```python
from build123d import *

# Parameters (mm, degrees)
BOSS_EXTRUDE1_DEPTH = 6.35
BOSS_EXTRUDE2_DEPTH = 6.35
CUT_EXTRUDE2_REACH  = 173.121
SKETCH3_R           = 25.4
SKETCH3_R_2         = 14.2875


with BuildPart() as part:
    # Sketch1 → Boss-Extrude1 (new body)
    with BuildSketch(Plane(origin=(0, 0, 0), x_dir=(1, 0, 0), z_dir=(0, 1, 0))):
        with BuildLine():
            Line((-82.55, -44.45), (-10.295626201, -144.494517568))
            ThreePointArc((-10.295626201, -144.494517568), (0, -149.758787534), (10.295626201, -144.494517568))
            Line((10.295626201, -144.494517568), (82.55, -44.45))
            Line((82.55, -44.45), (82.55, 44.45))
            Line((82.55, 44.45), (-82.55, 44.45))
            Line((-82.55, 44.45), (-82.55, -44.45))
        make_face()
    extrude(amount=BOSS_EXTRUDE1_DEPTH)

    # Sketch4 → Boss-Extrude2 (add)
    with BuildSketch(Plane(origin=(0, 6.35, 0), x_dir=(1, 0, 0), z_dir=(0, 1, 0))):
        Polygon((-63.5, -70.826923077), (-63.5, -96.226923077), (-57.15, -96.226923077), (-57.15, -79.619230769), align=None)
        Polygon((57.15, -96.226923077), (63.5, -96.226923077), (63.5, -70.826923077), (57.15, -79.619230769), align=None)
    extrude(amount=-BOSS_EXTRUDE2_DEPTH)

    # Sketch3 → Cut-Extrude2 (cut, up to next)
    with BuildSketch(Plane(origin=(0, 6.35, 0), x_dir=(1, 0, 0), z_dir=(0, 1, 0)), mode=Mode.PRIVATE) as cut_extrude2_sk1:
        with Locations(Location((0, -50.8, 0), (0, 0, 270))):
            Circle(SKETCH3_R)
    cut_extrude2_tool1 = extrude(cut_extrude2_sk1.sketch, amount=-CUT_EXTRUDE2_REACH, mode=Mode.PRIVATE) & part.part
    # Sketch3 → Cut-Extrude2 (cut, up to next)
    with BuildSketch(Plane(origin=(0, 6.35, 0), x_dir=(1, 0, 0), z_dir=(0, 1, 0)), mode=Mode.PRIVATE) as cut_extrude2_sk2:
        with Locations(Location((0, -120.65, 0), (0, 0, 270))):
            Circle(SKETCH3_R_2)
    cut_extrude2_tool2 = extrude(cut_extrude2_sk2.sketch, amount=-CUT_EXTRUDE2_REACH, mode=Mode.PRIVATE) & part.part
    # Sketch3 → Cut-Extrude2 (cut, up to next)
    with BuildSketch(Plane(origin=(0, 6.35, 0), x_dir=(1, 0, 0), z_dir=(0, 1, 0)), mode=Mode.PRIVATE) as cut_extrude2_sk3:
        with BuildLine():
            Line((-40.026450178, 28.764752129), (-8.690133469, 11.891350824))
            ThreePointArc((-8.690133469, 11.891350824), (-7.123451286, 11.92620437), (-6.35, 13.289098695))
            Line((-6.35, 13.289098695), (-6.35, 30.1625))
            ThreePointArc((-6.35, 30.1625), (-6.814967985, 31.285032015), (-7.9375, 31.75))
            Line((-7.9375, 31.75), (-39.273816708, 31.75))
            ThreePointArc((-39.273816708, 31.75), (-40.813147894, 30.550592453), (-40.026450178, 28.764752129))
        make_face()
    cut_extrude2_tool3 = extrude(cut_extrude2_sk3.sketch, amount=-CUT_EXTRUDE2_REACH, mode=Mode.PRIVATE) & part.part
    # Sketch3 → Cut-Extrude2 (cut, up to next)
    with BuildSketch(Plane(origin=(0, 6.35, 0), x_dir=(1, 0, 0), z_dir=(0, 1, 0)), mode=Mode.PRIVATE) as cut_extrude2_sk4:
        with BuildLine():
            Line((-69.85, 27.741670535), (-69.85, 7.9375))
            ThreePointArc((-69.85, 7.9375), (-69.385032015, 6.814967985), (-68.2625, 6.35))
            Line((-68.2625, 6.35), (-31.483326149, 6.35))
            ThreePointArc((-31.483326149, 6.35), (-29.943994963, 7.549407547), (-30.73069268, 9.335247871))
            Line((-30.73069268, 9.335247871), (-67.509866531, 29.139418406))
            ThreePointArc((-67.509866531, 29.139418406), (-69.076548714, 29.10456486), (-69.85, 27.741670535))
        make_face()
    cut_extrude2_tool4 = extrude(cut_extrude2_sk4.sketch, amount=-CUT_EXTRUDE2_REACH, mode=Mode.PRIVATE) & part.part
    # Sketch3 → Cut-Extrude2 (cut, up to next)
    with BuildSketch(Plane(origin=(0, 6.35, 0), x_dir=(1, 0, 0), z_dir=(0, 1, 0)), mode=Mode.PRIVATE) as cut_extrude2_sk5:
        with BuildLine():
            Line((7.9375, 31.75), (39.273816708, 31.75))
            ThreePointArc((39.273816708, 31.75), (40.813147894, 30.550592453), (40.026450178, 28.764752129))
            Line((40.026450178, 28.764752129), (8.690133469, 11.891350824))
            ThreePointArc((8.690133469, 11.891350824), (7.123451286, 11.92620437), (6.35, 13.289098695))
            Line((6.35, 13.289098695), (6.35, 30.1625))
            ThreePointArc((6.35, 30.1625), (6.814967985, 31.285032015), (7.9375, 31.75))
        make_face()
    cut_extrude2_tool5 = extrude(cut_extrude2_sk5.sketch, amount=-CUT_EXTRUDE2_REACH, mode=Mode.PRIVATE) & part.part
    # Sketch3 → Cut-Extrude2 (cut, up to next)
    with BuildSketch(Plane(origin=(0, 6.35, 0), x_dir=(1, 0, 0), z_dir=(0, 1, 0)), mode=Mode.PRIVATE) as cut_extrude2_sk6:
        with BuildLine():
            Line((30.73069268, 9.335247871), (67.509866531, 29.139418406))
            ThreePointArc((67.509866531, 29.139418406), (69.076548714, 29.10456486), (69.85, 27.741670535))
            Line((69.85, 27.741670535), (69.85, 7.9375))
            ThreePointArc((69.85, 7.9375), (69.385032015, 6.814967985), (68.2625, 6.35))
            Line((68.2625, 6.35), (31.483326149, 6.35))
            ThreePointArc((31.483326149, 6.35), (29.943994963, 7.549407547), (30.73069268, 9.335247871))
        make_face()
    cut_extrude2_tool6 = extrude(cut_extrude2_sk6.sketch, amount=-CUT_EXTRUDE2_REACH, mode=Mode.PRIVATE) & part.part
    # Sketch3 → Cut-Extrude2 (cut, up to next)
    with BuildSketch(Plane(origin=(0, 6.35, 0), x_dir=(1, 0, 0), z_dir=(0, 1, 0)), mode=Mode.PRIVATE) as cut_extrude2_sk7:
        with BuildLine():
            Line((69.85, -27.741670535), (69.85, -7.9375))
            ThreePointArc((69.85, -7.9375), (69.385032015, -6.814967985), (68.2625, -6.35))
            Line((68.2625, -6.35), (31.483326149, -6.35))
            ThreePointArc((31.483326149, -6.35), (29.943994963, -7.549407547), (30.73069268, -9.335247871))
            Line((30.73069268, -9.335247871), (67.509866531, -29.139418406))
            ThreePointArc((67.509866531, -29.139418406), (69.076548714, -29.10456486), (69.85, -27.741670535))
        make_face()
    cut_extrude2_tool7 = extrude(cut_extrude2_sk7.sketch, amount=-CUT_EXTRUDE2_REACH, mode=Mode.PRIVATE) & part.part
    # Sketch3 → Cut-Extrude2 (cut, up to next)
    with BuildSketch(Plane(origin=(0, 6.35, 0), x_dir=(1, 0, 0), z_dir=(0, 1, 0)), mode=Mode.PRIVATE) as cut_extrude2_sk8:
        with BuildLine():
            Line((-30.73069268, -9.335247871), (-67.509866531, -29.139418406))
            ThreePointArc((-67.509866531, -29.139418406), (-69.076548714, -29.10456486), (-69.85, -27.741670535))
            Line((-69.85, -27.741670535), (-69.85, -7.9375))
            ThreePointArc((-69.85, -7.9375), (-69.385032015, -6.814967985), (-68.2625, -6.35))
            Line((-68.2625, -6.35), (-31.483326149, -6.35))
            ThreePointArc((-31.483326149, -6.35), (-29.943994963, -7.549407547), (-30.73069268, -9.335247871))
        make_face()
    cut_extrude2_tool8 = extrude(cut_extrude2_sk8.sketch, amount=-CUT_EXTRUDE2_REACH, mode=Mode.PRIVATE) & part.part
    # Sketch3 → Cut-Extrude2 (cut, up to next)
    with BuildSketch(Plane(origin=(0, 6.35, 0), x_dir=(1, 0, 0), z_dir=(0, 1, 0)), mode=Mode.PRIVATE) as cut_extrude2_sk9:
        with BuildLine():
            Line((-6.35, -85.142875899), (-6.35, -99.265701316))
            ThreePointArc((-6.35, -99.265701316), (-15.402705776, -104.514096399), (-21.066111407, -113.313128703))
            Line((-21.066111407, -113.313128703), (-61.628371026, -57.15))
            Line((-61.628371026, -57.15), (-34.342875899, -57.15))
            ThreePointArc((-34.342875899, -57.15), (-24.695704333, -75.495704333), (-6.35, -85.142875899))
        make_face()
    cut_extrude2_tool9 = extrude(cut_extrude2_sk9.sketch, amount=-CUT_EXTRUDE2_REACH, mode=Mode.PRIVATE) & part.part
    # Sketch3 → Cut-Extrude2 (cut, up to next)
    with BuildSketch(Plane(origin=(0, 6.35, 0), x_dir=(1, 0, 0), z_dir=(0, 1, 0)), mode=Mode.PRIVATE) as cut_extrude2_sk10:
        with BuildLine():
            Line((6.35, -85.142875899), (6.35, -99.265701316))
            ThreePointArc((6.35, -99.265701316), (15.402705776, -104.514096399), (21.066111407, -113.313128703))
            Line((21.066111407, -113.313128703), (61.628371026, -57.15))
            Line((61.628371026, -57.15), (34.342875899, -57.15))
            ThreePointArc((34.342875899, -57.15), (24.695704333, -75.495704333), (6.35, -85.142875899))
        make_face()
    cut_extrude2_tool10 = extrude(cut_extrude2_sk10.sketch, amount=-CUT_EXTRUDE2_REACH, mode=Mode.PRIVATE) & part.part
    # Sketch3 → Cut-Extrude2 (cut, up to next)
    with BuildSketch(Plane(origin=(0, 6.35, 0), x_dir=(1, 0, 0), z_dir=(0, 1, 0)), mode=Mode.PRIVATE) as cut_extrude2_sk11:
        with BuildLine():
            Line((-19.05, -21.527946348), (-19.05, 0))
            ThreePointArc((-19.05, 0), (0, 5.652946348), (19.05, 0))
            Line((19.05, 0), (19.05, -21.527946348))
            ThreePointArc((19.05, -21.527946348), (0, -15.875), (-19.05, -21.527946348))
        make_face()
    cut_extrude2_tool11 = extrude(cut_extrude2_sk11.sketch, amount=-CUT_EXTRUDE2_REACH, mode=Mode.PRIVATE) & part.part
    # Sketch3 → Cut-Extrude2 (cut, up to next)
    with BuildSketch(Plane(origin=(0, 6.35, 0), x_dir=(1, 0, 0), z_dir=(0, 1, 0)), mode=Mode.PRIVATE) as cut_extrude2_sk12:
        with BuildLine():
            Line((-62.859530994, -44.45), (-35.639286609, -44.45))
            ThreePointArc((-35.639286609, -44.45), (-34.646236712, -44.101050827), (-34.089752409, -43.207608696))
            ThreePointArc((-34.089752409, -43.207608696), (-32.045675665, -36.913665127), (-28.851086957, -31.11827227))
            ThreePointArc((-28.851086957, -31.11827227), (-28.645591226, -30.691776493), (-28.575, -30.223648283))
            Line((-28.575, -30.223648283), (-28.575, -25.256406388))
            ThreePointArc((-28.575, -25.256406388), (-29.348451286, -23.893512063), (-30.915133469, -23.858658517))
            Line((-30.915133469, -23.858658517), (-63.612164463, -41.464752129))
            ThreePointArc((-63.612164463, -41.464752129), (-64.398862179, -43.250592453), (-62.859530994, -44.45))
        make_face()
    cut_extrude2_tool12 = extrude(cut_extrude2_sk12.sketch, amount=-CUT_EXTRUDE2_REACH, mode=Mode.PRIVATE) & part.part
    # Sketch3 → Cut-Extrude2 (cut, up to next)
    with BuildSketch(Plane(origin=(0, 6.35, 0), x_dir=(1, 0, 0), z_dir=(0, 1, 0)), mode=Mode.PRIVATE) as cut_extrude2_sk13:
        with BuildLine():
            Line((28.575, -25.256406388), (28.575, -30.223648283))
            ThreePointArc((28.575, -30.223648283), (28.645591226, -30.691776493), (28.851086957, -31.11827227))
            ThreePointArc((28.851086957, -31.11827227), (32.045675665, -36.913665127), (34.089752409, -43.207608696))
            ThreePointArc((34.089752409, -43.207608696), (34.646236712, -44.101050827), (35.639286609, -44.45))
            Line((35.639286609, -44.45), (62.859530994, -44.45))
            ThreePointArc((62.859530994, -44.45), (64.398862179, -43.250592453), (63.612164463, -41.464752129))
            Line((63.612164463, -41.464752129), (30.915133469, -23.858658517))
            ThreePointArc((30.915133469, -23.858658517), (29.348451286, -23.893512063), (28.575, -25.256406388))
        make_face()
    cut_extrude2_tool13 = extrude(cut_extrude2_sk13.sketch, amount=-CUT_EXTRUDE2_REACH, mode=Mode.PRIVATE) & part.part
    add(cut_extrude2_tool1.solids().sort_by_distance((0, 6.35, 50.8))[0], mode=Mode.SUBTRACT)
    add(cut_extrude2_tool2.solids().sort_by_distance((0, 6.35, 120.65))[0], mode=Mode.SUBTRACT)
    add(cut_extrude2_tool3.solids().sort_by_distance((-19.115543, 6.35, -24.652033))[0], mode=Mode.SUBTRACT)
    add(cut_extrude2_tool4.solids().sort_by_distance((-55.236845, 6.35, -14.418636))[0], mode=Mode.SUBTRACT)
    add(cut_extrude2_tool5.solids().sort_by_distance((19.115543, 6.35, -24.652033))[0], mode=Mode.SUBTRACT)
    add(cut_extrude2_tool6.solids().sort_by_distance((55.236845, 6.35, -14.418636))[0], mode=Mode.SUBTRACT)
    add(cut_extrude2_tool7.solids().sort_by_distance((55.236845, 6.35, 14.418636))[0], mode=Mode.SUBTRACT)
    add(cut_extrude2_tool8.solids().sort_by_distance((-55.236845, 6.35, 14.418636))[0], mode=Mode.SUBTRACT)
    add(cut_extrude2_tool9.solids().sort_by_distance((-30.896348, 6.35, 81.78683))[0], mode=Mode.SUBTRACT)
    add(cut_extrude2_tool10.solids().sort_by_distance((30.896348, 6.35, 81.78683))[0], mode=Mode.SUBTRACT)
    add(cut_extrude2_tool11.solids().sort_by_distance((0, 6.35, 6.929783))[0], mode=Mode.SUBTRACT)
    add(cut_extrude2_tool12.solids().sort_by_distance((-43.155831, 6.35, 36.82378))[0], mode=Mode.SUBTRACT)
    add(cut_extrude2_tool13.solids().sort_by_distance((43.155831, 6.35, 36.82378))[0], mode=Mode.SUBTRACT)


solid = part.part
```
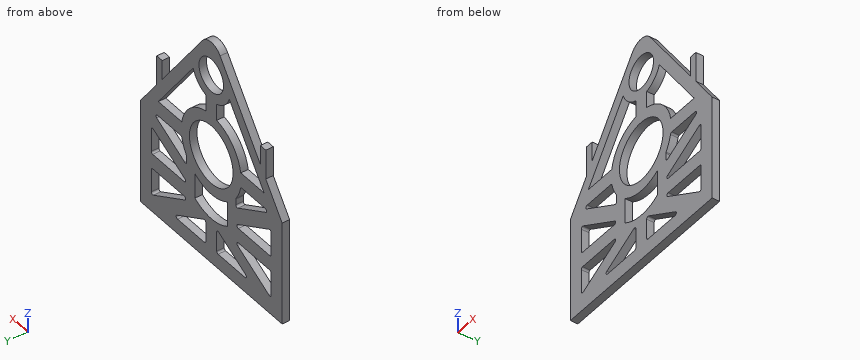
Input: part model. Units: mm. Frame: model coordinates. Round coordinates to 2 decimals unless told otherwise and drop trailing zeros. Write each loop counter-clockwise with the first axis right and the second up, starting at its lowest first coordinate (ties: lowest second). Pieces come first, ordered by that corner, then holes. Notation, with made-up numbers: (-28, 57) -> (26, 57) arc R28 ccw to (26, 94) -> close; hole circle Ø2 at (50.25, 43.25). An arc over 180 degrees is marked (long way). Answer as CSV lines item,"result".
1. Ray query, L1, parallel to Z at x = 69.5, y = 0.5; L2, parallel to X at y = 1.75, z = -6.5; L3, parallel to Z at x = 7, y = 3.75. Return the intervals inside material, ascending. Write a range as [from, to].
Geometry says:
L1,"z = [-44.45, -28.74], [-6.94, 6.94], [28.74, 62.52]"
L2,"x = [-82.55, -68.94], [-30.81, 30.81], [68.94, 82.55]"
L3,"z = [-44.45, -31.44], [-12.01, -4.94], [16.58, 26.38], [75.22, 85.02], [99.47, 108.19], [133.11, 147.66]"
2. Contact query for a flat-ended pin moving along its axis: P1, Ø3, axis at x = -18, y = 1.5, coming from the +Z side. Output: stop coordinate, or through.
Geometry says:
P1,"stops at z = 135.9"
3. Section B-B (x = -44). Return the cut outline in (y, z), plus the area to 3 significant figures.
Geometry says:
outline,"(0, -44.45) -> (6.35, -44.45) -> (6.35, -16.48) -> (0, -16.48) -> close; (0, -6.35) -> (6.35, -6.35) -> (6.35, 6.35) -> (0, 6.35) -> close; (0, 16.48) -> (6.35, 16.48) -> (6.35, 30.9) -> (0, 30.9) -> close; (0, 44.45) -> (6.35, 44.45) -> (6.35, 57.15) -> (0, 57.15) -> close; (0, 81.56) -> (6.35, 81.56) -> (6.35, 97.83) -> (0, 97.83) -> close"
area,"534 mm^2"
4. Section A-A (x = 0). Give the number of separate pieces and of enclosed holes in the cut face, plus the area to 3 significant figures.
Geometry says:
separate pieces,"4"
enclosed holes,"0"
area,"592 mm^2"
5. Section C-C (z = 126.5). Return the cut outline in (x, y).
Geometry says:
outline,"(-23.29, 0) -> (-13.03, 0) -> (-13.03, 6.35) -> (-23.29, 6.35) -> close; (13.03, 0) -> (23.29, 0) -> (23.29, 6.35) -> (13.03, 6.35) -> close"
